Geometry: final body of the model. Coordinates: model frame, mm. Face numbers are marked on the shaded views. A direction names the side the tool comes from. Round coordinates to 2 decimals unless told otherwise and drop trailing zeros. Write each loop counter-clockwise with the first axis right and the second up, starting at its lowest first coordinate (ties: lowest second). Pieces come first, ordered by that corner, then holes. Notation, with made-up numbers: M 43,-27.75 L 72,-27.75 A27 ccw 72,2.25 Z; hole C 25.25,-14 d8. An arc over 180 degrees is marked long. Answer as CSV lines item,"result". Start each with the question number.
Q1. Section query D-D on z = 50.5. Output: boundary loops of the cut face in (x, y), and give its area (3 significant figures).
Q2. Mould query, pull axis Z, two halves, no side actions, for the marked faces 1, 2 and 3. Classes: pulls with the +Z half, pulls with the -Z half, needs draft (parallel to the pull), parting line crosses it, or undercut.
Q3. Ray query, probe 1 along X at (y, z) = (21, 28); probe 2 along X at (y, z) = (18.5, 35.5); probe 3 along Z at (x, y) = (27.5, 25.75). Return the intervals inside material, ascending.
Q4. Section query C-C on z = 35.5. Output: boundary loops of the cut face in (x, y), and give its area (3 significant figures).
Q5. Section query B-B on y = 16. Output: boundary loops of the cut face in (x, z), and give its area (3 significant figures).
Q6. Section query A-A on x = 45.5. Output: boundary loops of the cut face in (y, z), and give its area (3 significant figures).
Q7. Reachability of the marked faces 4 and 5 from +Z, -Z, +X, -X, +Y, -Y: full face, straight path, thin tool, end or side. Return the list, or none.
Q8. First-contact query: pin 1 (1.5 mm diameter, centred on y = 22.5, z = 48.5, fed in from -X). Flat tip, straight axial feed; report the tip coordinate or a pass-through.
```python
from build123d import *

# Parameters (mm, degrees)
F0_W     = 40.132
F0_H     = 19.05
F1_DEPTH = 62.23
F3_DEPTH = 25.4
F5_DEPTH = 25.4


with BuildPart() as f1:
    # F0 (on Top) → F1 (new body)
    with BuildSketch(Plane.XY):
        with Locations((34.380583, 22.322809)):
            Rectangle(F0_W, F0_H)
    extrude(amount=F1_DEPTH)

    # F2 (on face) → F3 (cut)
    with BuildSketch(Plane.XZ.offset(-12.797809)):
        Polygon((49.35965, 29.470933), (34.380583, 44.45), (34.380583, 29.470933), align=None)
        Polygon((34.380583, 29.470933), (34.380583, 44.45), (19.385723, 29.470933), align=None)
        with BuildLine():
            Line((49.35965, 29.470933), (34.380583, 29.470933))
            Line((34.380583, 29.470933), (34.380583, 5.267071))
            ThreePointArc((34.380583, 5.267071), (38.556777, 8.086362), (37.500633, 13.013183))
            Line((37.500633, 13.013183), (49.35965, 27.438933))
            Line((49.35965, 27.438933), (49.35965, 29.470933))
        make_face()
        with BuildLine():
            Line((34.380583, 5.267071), (34.380583, 29.470933))
            Line((34.380583, 29.470933), (19.385723, 29.470933))
            Line((19.385723, 29.470933), (19.385723, 27.438933))
            Line((19.385723, 27.438933), (31.262963, 13.013183))
            ThreePointArc((31.262963, 13.013183), (30.206365, 8.087489), (34.380583, 5.267071))
        make_face()
    extrude(amount=-F3_DEPTH, mode=Mode.SUBTRACT)

    # F4 (on face) → F5 (cut)
    with BuildSketch(Plane.XZ.offset(-12.797809)):
        Polygon((14.314583, 62.23), (14.314583, 30.48), (24.220583, 62.23), align=None)
        Polygon((54.446583, 62.23), (44.540583, 62.23), (54.446583, 30.48), align=None)
    extrude(amount=-F5_DEPTH, mode=Mode.SUBTRACT)


solid = f1.part
```
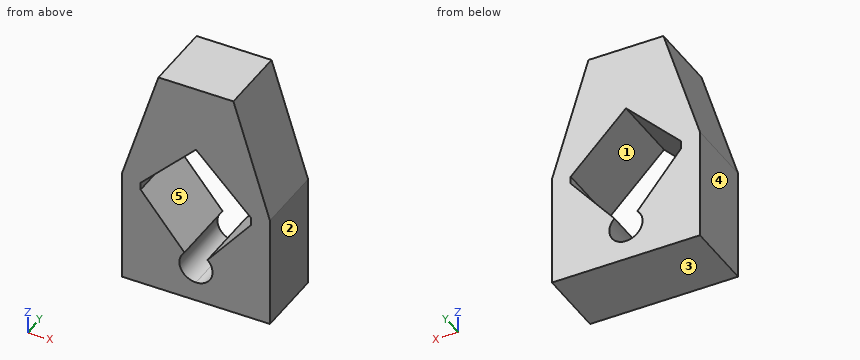
Entries:
1,outline,"M 20.56,12.8 L 48.2,12.8 L 48.2,31.85 L 20.56,31.85 Z"
1,area,"527 mm^2"
2,face 1,"undercut"
2,face 2,"needs draft"
2,face 3,"pulls with the -Z half"
3,probe 1,"x = 14.31 to 19.39, 49.36 to 54.45"
3,probe 2,"x = 15.88 to 25.42, 43.33 to 52.88"
3,probe 3,"z = 0 to 17.58, 37.58 to 62.23"
4,outline,"M 15.88,12.8 L 25.42,12.8 L 25.42,31.85 L 15.88,31.85 Z; M 43.33,12.8 L 52.88,12.8 L 52.88,31.85 L 43.33,31.85 Z"
4,area,"364 mm^2"
5,outline,"M 14.31,0 L 54.45,0 L 54.45,30.48 L 44.54,62.23 L 24.22,62.23 L 14.31,30.48 Z; hole M 19.39,27.44 L 31.26,13.01 A4.5 ccw long 37.5,13.01 L 49.36,27.44 L 49.36,29.47 L 34.38,44.45 L 19.39,29.47 Z"
5,area,"1,580 mm^2"
6,outline,"M 12.8,0 L 31.85,0 L 31.85,22.74 L 12.8,22.74 Z; M 12.8,33.33 L 31.85,33.33 L 31.85,59.15 L 12.8,59.15 Z"
6,area,"925 mm^2"
7,face 4,"+Z, -Z, -X, +Y, -Y"
7,face 5,"+Y, -Y"
8,pin 1,"stops at x = 19.7"
